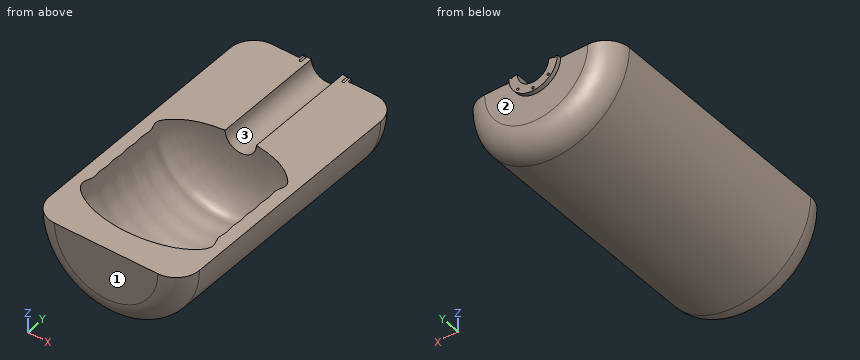
Autodesk Inventor part; units mm, degrees
ref_plane "YZ Plane" through (0, 0, 0) normal (1, 0, 0) x (0, 1, 0)
ref_plane "XZ Plane" through (0, 0, 0) normal (0, 1, 0) x (-1, 0, 0)
ref_plane "XY Plane" through (0, 0, 0) normal (0, 0, 1) x (1, 0, 0)
sketch "InnerShape" plane through (0, 0, 0) normal (0, 0, 1) x (1, 0, 0)
  spline S0 degree 4 poles (25.5438, 42.0281) (88.3985, 41.1205) (175.7883, 56.4516) (240.2524, 85.3572) (289.1446, 125.5476) (307.0428, 154.2136) (298.3402, 181.4897) (286.4701, 206.6436) (294.5788, 232.4697) (293.8632, 257.9202) (288.0995, 283.3382) (294.0239, 308.6783) (294.0576, 334.1754) (288.0277, 359.5276) (294.0484, 384.8821) (294.0529, 410.3743) (288.018, 435.7273) (294.0857, 461.094) (293.9522, 486.6266) (288.2436, 512.1618) (293.3771, 538.0681) (309.1971, 564.4637) (288.3219, 593.5581) (240.7199, 632.9003) (183.1395, 665.8542) (80.5578, 674.6739) (25.5438, 677.0281) knots 0 0 0 0 0 0.143858 0.187431 0.224823 0.259091 0.291676 0.323874 0.356024 0.388045 0.420047 0.452068 0.484088 0.516091 0.548112 0.580132 0.612135 0.644156 0.676226 0.708422 0.741006 0.775272 0.812434 0.855963 1 1 1 1 1
  point P0 (254.729, 359.5281)
  point P1 (142.9438, 54.7281)
  point P2 (219.4438, 80.1281)
  point P3 (263.0438, 105.5281)
  point P4 (290.4438, 130.9281)
  point P5 (302.0438, 156.3281)
  point P6 (297.4438, 181.7281)
  point P7 (290.4438, 207.1281)
  point P8 (292.8438, 232.5281)
  point P9 (292.8438, 257.9281)
  point P10 (290.4438, 283.3281)
  point P11 (292.8438, 308.7281)
  point P12 (292.8438, 334.1281)
  point P13 (290.4438, 359.5281)
  point P14 (292.8438, 384.9281)
  point P15 (292.8438, 410.3281)
  point P16 (290.4438, 435.7281)
  point P17 (292.8438, 461.1281)
  point P18 (292.8438, 486.5281)
  point P19 (290.4438, 511.9281)
  point P20 (295.1438, 537.3281)
  point P21 (302.0438, 562.7281)
  point P22 (290.4438, 588.1281)
  point P23 (263.0438, 613.5281)
  point P24 (222.6438, 638.9281)
  point P25 (142.9438, 664.3281)
sketch "Sketch2" plane through (0, 0, 0) normal (0, 0, 1) x (1, 0, 0)
  line L0 (66.5, 630.0055) -> (66.5, 1106)
  line L1 (66.5, 1106) -> (103.5, 1106)
  line L2 (103.5, 1106) -> (103.5, 1088)
  line L3 (103.5, 1088) -> (220, 1088)
  line L4 (320, 988) -> (320, -12)
  line L5 (220, -112) -> (0, -112)
  line L6 (0, -112) -> (0, 0)
  arc A0 (320, 988) -> (220, 1088) centre (220, 988) ccw
  arc A1 (220, -112) -> (320, -12) centre (220, -12) ccw
  spline S0 degree 4 poles (0, 0) (62.8547, -0.9075) (150.2445, 14.4235) (214.7086, 43.3291) (263.6008, 83.5195) (281.499, 112.1856) (272.7964, 139.4616) (260.9263, 164.6155) (269.035, 190.4417) (268.3194, 215.8922) (262.5557, 241.3102) (268.4801, 266.6503) (268.5138, 292.1474) (262.4839, 317.4996) (268.5046, 342.854) (268.5091, 368.3463) (262.4742, 393.6993) (268.5419, 419.0659) (268.4084, 444.5985) (262.6998, 470.1338) (267.8333, 496.04) (283.6534, 522.4356) (262.7781, 551.5301) (215.1761, 590.8722) (157.5957, 623.8262) (55.014, 632.6458) (0, 635) knots 0 0 0 0 0 0.143858 0.187431 0.224823 0.259091 0.291676 0.323874 0.356024 0.388045 0.420047 0.452068 0.484088 0.516091 0.548112 0.580132 0.612135 0.644156 0.676226 0.708422 0.741006 0.775272 0.812434 0.855963 1 1 1 1 1
  point P0 (320, 1088)
  point P1 (320, -112)
  point P2 (0, 0)
  dimension "d9" = 1106
  dimension "d10" = 66.5
  dimension "d11" = 103.5
  dimension "d12" = 320
  dimension "d13" = 18
  dimension "d14" = 1200
  dimension "d15" = 100
  dimension "d16" = 100
revolve "Revolution1" add sketch "Sketch2" angle 360 about axis through (0, -112, 0) along (0, 1, 0)
sketch "Sketch3" plane through (0, 1106, 0) normal (0, 1, 0) x (1, 0, 0)
  point P0 (0, 0)
  point P1 (0, 91)
  dimension "d18" = 91
hole "Hole1" at (0, 1106, -91) direction (0, -1, 0) diameter 10.106 depth 30 tip angle 118
pattern_circular "Circular Pattern1" count 8 over 360 about axis through (0, 868.0028, 0) along (0, 1, 0) of "Hole1"
sketch "Sketch5" plane through (0, 1106, 0) normal (0, 1, 0) x (1, 0, 0)
  circle A0 centre (0, 0) radius 320
  line L0 (-320, 0) -> (320, 0)
  line L1 (320, 0) -> (320, -320)
  line L2 (320, -320) -> (-320, -320)
  line L3 (-320, -320) -> (-320, 0)
  point P0 (0, -320)
extrude "Extrusion2" cut sketch "Sketch5" against normal through all contours A0 L0 | A0 L2 L3 picked at (-65.063, -184.508)
properties part number "TransportDewar"
Could you check a few things on this model? Use its own coordinates, in mm. Face numbers are marked on the shaded views. A direction names the side the tool comes from. Round coordinates to 2 decimals unless told otherwise and drop trailing zeros. Order: outer loops, then holes, each group sorted by start corner. A loop starts at its lowest first (then second) coordinate and runs counter-clockwise, first axis right, second up. Notation, with made-up numbers: M -18,58.5 L 32,58.5 A11 cw 32,64.5 Z; hole C 84,-27 d7. An arc over 180 degrees is marked long. One line per question, with ' | ' between items. Start each with the question number.
(1) For P1, Ø12, axis at y = 367.5, z = -138.5, coming from the -X side; P2, Ø1, axis at y = 367, z = -227.5, coming from the +X side; P3, Ø3, axis at y = 421, z = -93.5, coming from the +X side, each with a flat end and sliding along its axis, tell me the tip position at first contact or that it passes through.
(2) Suppose I cut it at A-A on y = 1011. List the corners of the cut face in (x, z) for me.
(3) Please list where these lines run through material, in increasing order: line 1 along Z through (x, y) = (0, 1099); line 2 along X through (y, z) = (144.5, -144); line 3 along X through (y, z) = (1093.5, -91).
(4) For the marked faces 1, 2 and 3, which set-ups out of +Z, -Z, +X, -X, +Y, -Y let a thin tool reach every point of the face, with its end or its side?
Geometry results:
1) P1: x = -291.28 | P2: x = 225.55 | P3: x = 306.49
2) outline: M -317.32,0 A317.32 ccw 317.32,0 L 66.5,0 A66.5 cw -66.5,0 Z
3) line 1: -103.5 to -96.05, -85.95 to -66.5 | line 2: -285.77 to -228.56, 228.56 to 285.77 | line 3: -49.31 to -5.05, 5.05 to 49.31
4) face 1: +Z, -Z, +X, -X, -Y | face 2: -Z, +Y | face 3: +Z, +Y
